Answer from the drawing. Dimensions are ordinates in mm from the lowest x, y and z of the part. Give positions to 0.01 mm unless a question says otherwise; leave off trailing zeros. Write each loop counter-clockwise with the first axis right and the second up, starting at its lowest first coordinate (ties: lowest second). Pieces come first, ordered by that corner, then holes. Notation, with made-up numbers: M 74.5,-24.5 L 112.5,-24.5 A16 ccw 112.5,-16.5 Z; hole C 75.5,85 d8. An arc over 180 degrees is marked long. Answer as a JSON object with one key per item and string values.
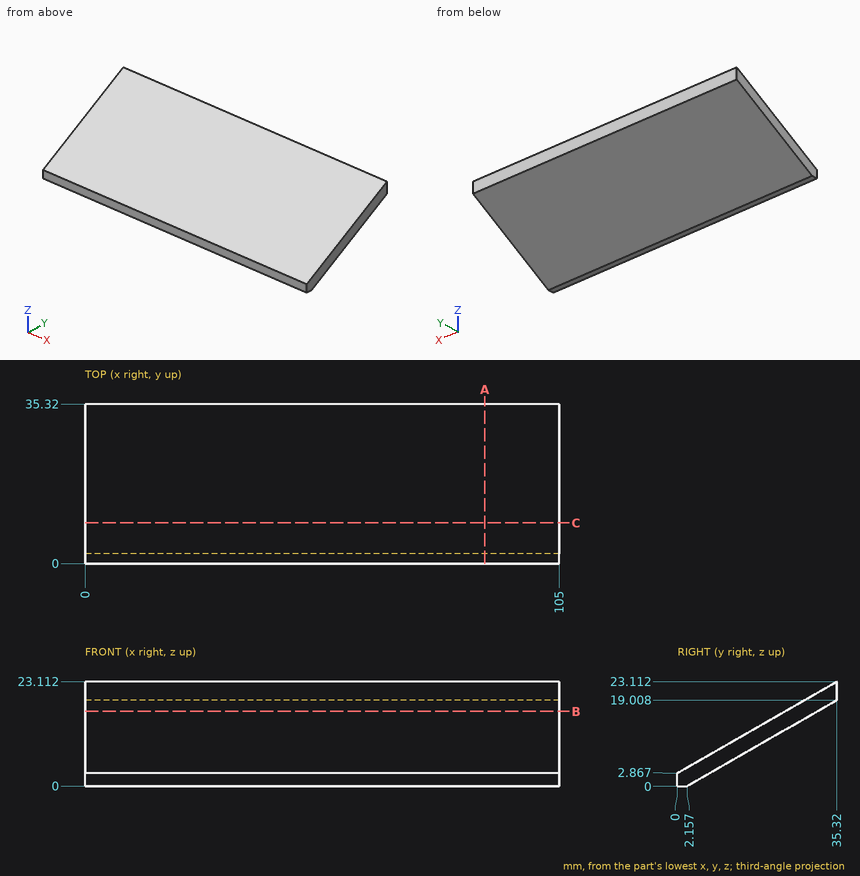
1. A cutting plane is placed at B-B, the plane z = 16.5. Give the vertices of the cut face in (x, y) (1 decimal).
Verdict:
{"outline": "M 0,23.8 L 105,23.8 L 105,30.9 L 0,30.9 Z"}
2. A cutting plane is placed at A-A, the plane x = 88.5. Give the vertices of the cut face in (y, z).
Verdict:
{"outline": "M 0,0 L 2.16,0 L 35.32,19.01 L 35.32,23.11 L 0,2.87 Z"}
3. A cutting plane is placed at C-C, the plane y = 9. Give the vertices of the cut face in (x, z), plus the area to 3 significant figures.
Verdict:
{"outline": "M 0,3.92 L 105,3.92 L 105,8.03 L 0,8.03 Z", "area": "431 mm2"}
4. Flat-ended cylindrical pins translate along their axes: pin 1 (12 mm diameter, centred on x = 79, z = 4, fed in from +Y) (1 decimal); pin 2 (10 mm diameter, centred on y = 26.5, z = 3, fed in from -X); pin 3 (4 mm diameter, centred on x = 90.5, y = 8, fed in from -Z). Find the tip coordinate at first contact, or state that the pin passes through.
Verdict:
{"pin 1": "stops at y = 19.6", "pin 2": "passes through", "pin 3": "stops at z = 2.2"}
5. Consider line 1 along Y through (x, z) = (23.5, 12.5) (1 decimal); line 2 along Y through (x, z) = (8, 19.5); line 3 along Z through (x, y) = (94, 9) (1 decimal). Determine where each line is inside the solid, lowest interval first.
Verdict:
{"line 1": "y = 16.8 to 24", "line 2": "y = 29.02 to 35.32", "line 3": "z = 3.9 to 8"}
